from build123d import *

# Parameters (mm, degrees)
SALIENTE_EXTRUIR1_DEPTH = 6
CROQUIS3_R              = 2
CORTAR_EXTRUIR1_DEPTH   = 33.186953879
CROQUIS5_R              = 5
CORTAR_EXTRUIR2_DEPTH   = 32.176914536


with BuildPart() as part:
    # Croquis2 → Saliente-Extruir1 (new, symmetric)
    with BuildSketch(Plane.XY):
        Polygon((0, 0), (0, 30), (2.5, 30), (10, 0), align=None)
    extrude(amount=SALIENTE_EXTRUIR1_DEPTH, both=True)

    # Croquis3 → Cortar-Extruir1 (cut, through all)
    with BuildSketch(Plane.ZY):
        with Locations((0, 20)):
            Circle(CROQUIS3_R)
    extrude(amount=-CORTAR_EXTRUIR1_DEPTH, mode=Mode.SUBTRACT)

    # Croquis5 → Cortar-Extruir2 (cut, through all)
    with BuildSketch(Plane.ZY.offset(-4)):
        with Locations((0, 20)):
            Circle(CROQUIS5_R)
    extrude(amount=-CORTAR_EXTRUIR2_DEPTH, mode=Mode.SUBTRACT)


solid = part.part
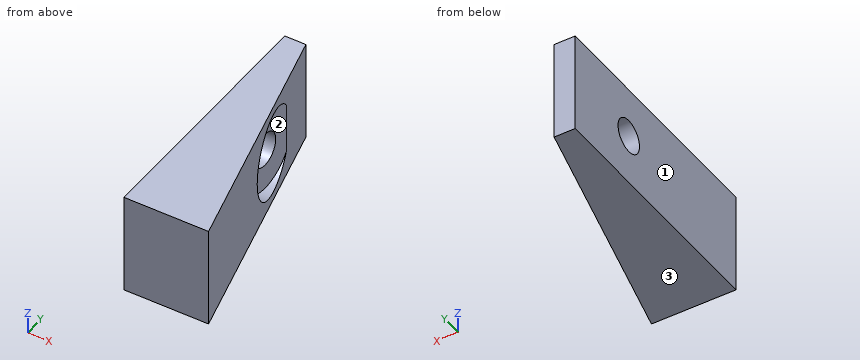
For this review, take the finished solid that the model builds, in its own axes (mm). Face numbers are marked on the shaded views. Coordinates: 2 decimals unless noted, no trailing zeros. Loops run counter-clockwise (first coordinate to the right, second up) from the corner with the lowest first, then second, coordinate; pieces in that order, holes last. Notation, with made-up numbers: (5.5, 38.5) - (46.5, 38.5) arc R21 cw to (46.5, 44.5) - close; hole circle Ø1 at (-1.75, 18). An arc over 180 degrees is marked (long way). Use a Markdown table: item, result. Add a question column.
Item 1: For line 1 (Z direction, x = 4.7, y = 20); line 2 (Y direction, x = 1.8, z = 0); line 3 (X direction, y = 20.5, z = 4.25), list the stretches that pass through material, from the lowest coordinate up.
Item 2: We need section D-D (y = 17). Give the boundary of the cut face in (x, z).
Item 3: Mouldability with a two-part tool opening along Z and no side actions: class the marked faces 1, 2 and 3 as pulls with the +Z half, pulls with the -Z half, needs draft (parallel to the pull), parting line crosses it, or undercut.
Item 4: We need section B-B (y = 20). Give the boundary of the cut face in (x, z).
Item 5: We need section A-A (z = 0). Give the boundary of the cut face in (x, y).
Item 6: We need section C-C (x = 2). Give the boundary of the cut face in (y, z), and give its area (3 significant figures).
Item 7: Insertion check: pin 1 Ø5 at (y, z) = (3.5, 4) entering from +X; pin 2 Ø2 at (x, z) = (5.5, 2.5) entering from +Y; pin 3 Ø2.5 at (y, z) = (21.5, -1.5) entering from +X. Each pin has a flat end and moves straight along its axis. Give the tip position at first contact, or say it passes through.
Results list:
| question | item | result |
|---|---|---|
| 1 | line 1 | z = -6 to -5, 5 to 6 |
| 1 | line 2 | y = 0 to 18, 22 to 30 |
| 1 | line 3 | x = 0 to 4 |
| 2 | outline | (0, -6) - (5.75, -6) - (5.75, -4) - (4, -4) - (4, 4) - (5.75, 4) - (5.75, 6) - (0, 6) - close |
| 3 | face 1 | needs draft |
| 3 | face 2 | undercut |
| 3 | face 3 | pulls with the -Z half |
| 4 | outline | (0, -6) - (5, -6) - (5, -5) - (4, -5) - (4, -2) - (0, -2) - close; (0, 2) - (4, 2) - (4, 5) - (5, 5) - (5, 6) - (0, 6) - close |
| 5 | outline | (0, 0) - (10, 0) - (6.25, 15) - (4, 15) - (4, 18) - (0, 18) - close; (0, 22) - (4, 22) - (4, 24) - (2.5, 30) - (0, 30) - close |
| 6 | outline | (0, -6) - (30, -6) - (30, 6) - (0, 6) - close; hole circle Ø4 at (20, 0) |
| 6 | area | 347 mm^2 |
| 7 | pin 1 | stops at x = 9.75 |
| 7 | pin 2 | stops at y = 16.43 |
| 7 | pin 3 | stops at x = 4 |
